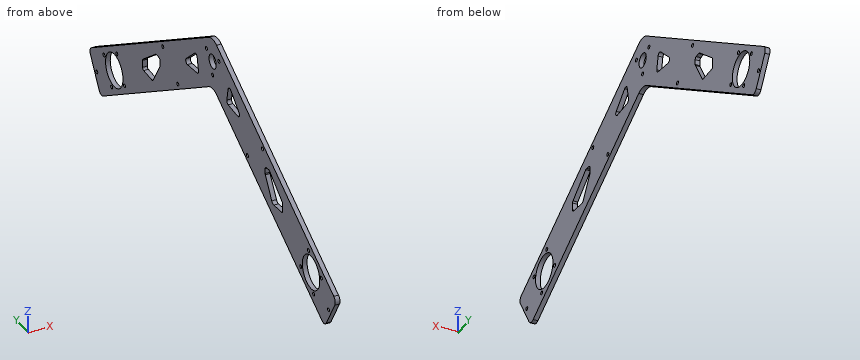
```python
from build123d import *

# Parameters (mm, degrees)
EXTRUDE_BASE_DEPTH         = 3.18
SKETCH4_R                  = 11.5
CUT_MOTOR_HOLES_DEPTH      = 3.18
SKETCH5_R                  = 1.25
MOTOR_SUPPORT_HOLES_DEPTH  = 3.18
SKETCH6_R                  = 1.25
SKETCH6_R_2                = 4.765
SUPPORT_HOLES_DEPTH        = 3.18
CUT_LIGHTENING_HOLES_DEPTH = 3.18


with BuildPart() as part:
    # bogie base → extrude-base (new body)
    with BuildSketch(Plane.YZ):
        with BuildLine():
            Line((-31.39506552, -5.945574909), (-20.11035906, -24.830897255))
            ThreePointArc((-20.11035906, -24.830897255), (-17.653836276, -26.657938255), (-14.624899277, -26.212827416))
            Line((-14.624899277, -26.212827416), (124.870587973, 57.141091427))
            ThreePointArc((124.870587973, 57.141091427), (130, 58.556853997), (135.129412027, 57.141091427))
            Line((135.129412027, 57.141091427), (274.624899277, -26.212827416))
            ThreePointArc((274.624899277, -26.212827416), (277.653836276, -26.657938255), (280.11035906, -24.830897255))
            Line((280.11035906, -24.830897255), (291.39506552, -5.945574909))
            ThreePointArc((291.39506552, -5.945574909), (291.840176358, -2.91663791), (290.013135359, -0.460115126))
            Line((290.013135359, -0.460115126), (135.129412027, 92.088866631))
            ThreePointArc((135.129412027, 92.088866631), (130, 93.504629201), (124.870587973, 92.088866631))
            Line((124.870587973, 92.088866631), (-30.013135359, -0.460115126))
            ThreePointArc((-30.013135359, -0.460115126), (-31.840176358, -2.91663791), (-31.39506552, -5.945574909))
        make_face()
    extrude(amount=EXTRUDE_BASE_DEPTH)

    # Sketch4 → Cut-motor holes (cut)
    with BuildSketch(Plane.YZ):
        with Locations((260, 0)):
            Circle(SKETCH4_R)
        Circle(SKETCH4_R)
    extrude(amount=CUT_MOTOR_HOLES_DEPTH, mode=Mode.SUBTRACT)

    # Sketch5 → motor support holes (cut)
    with BuildSketch(Plane.YZ):
        with Locations((3.419410151, 13.575994778)):
            Circle(SKETCH5_R)
        with Locations((-3.41941001, -13.575994814)):
            Circle(SKETCH5_R)
        with Locations((13.577380102, -3.419759)):
            Circle(SKETCH5_R)
        with Locations((-13.57737996, 3.419758964)):
            Circle(SKETCH5_R)
        with Locations((273.57737996, 3.419758964)):
            Circle(SKETCH5_R)
        with Locations((246.422619898, -3.419759)):
            Circle(SKETCH5_R)
        with Locations((263.41941001, -13.575994814)):
            Circle(SKETCH5_R)
        with Locations((256.580589849, 13.575994778)):
            Circle(SKETCH5_R)
    extrude(amount=MOTOR_SUPPORT_HOLES_DEPTH, mode=Mode.SUBTRACT)

    # Sketch6 → support holes (cut)
    with BuildSketch(Plane.YZ):
        with Locations((64.164835578, 52.110380567)):
            Circle(SKETCH6_R)
        with Locations((84.016579298, 36.433714107)):
            Circle(SKETCH6_R)
        with Locations((130, 77.68)):
            Circle(SKETCH6_R_2)
        with Locations((130, 68.17)):
            Circle(SKETCH6_R)
        with Locations((121.77231361, 82.449200841)):
            Circle(SKETCH6_R)
        with Locations((138.248750332, 82.43704307)):
            Circle(SKETCH6_R)
        with Locations((175.983420702, 36.433714107)):
            Circle(SKETCH6_R)
        with Locations((195.835164422, 52.110380567)):
            Circle(SKETCH6_R)
        with Locations((-23.022924787, -13.757083057)):
            Circle(SKETCH6_R)
        with Locations((283.022924787, -13.757083057)):
            Circle(SKETCH6_R)
    extrude(amount=SUPPORT_HOLES_DEPTH, mode=Mode.SUBTRACT)

    # Sketch7 → Cut-lightening holes (cut)
    with BuildSketch(Plane.YZ):
        with BuildLine():
            Line((54.884000108, 41.646401467), (38.03439682, 28.860792879))
            ThreePointArc((38.03439682, 28.860792879), (37.597600164, 28.332915929), (37.441118366, 27.665863577))
            Line((37.441118366, 27.665863577), (37.441118366, 22.734591544))
            ThreePointArc((37.441118366, 22.734591544), (37.849837551, 21.705462697), (38.853259944, 21.237166789))
            Line((38.853259944, 21.237166789), (49.165938422, 20.63209087))
            ThreePointArc((49.165938422, 20.63209087), (50.727348318, 20.966140733), (51.896208282, 22.053962665))
            Line((51.896208282, 22.053962665), (60.398420976, 35.861757183))
            ThreePointArc((60.398420976, 35.861757183), (60.564389902, 36.239537563), (60.621144468, 36.64824604))
            Line((60.621144468, 36.64824604), (60.621144468, 40.036157787))
            ThreePointArc((60.621144468, 40.036157787), (60.245516663, 41.02902594), (59.306761578, 41.524628912))
            Line((59.306761578, 41.524628912), (55.976338764, 41.939943289))
            ThreePointArc((55.976338764, 41.939943289), (55.401440776, 41.900078528), (54.884000108, 41.646401467))
        make_face()
        with BuildLine():
            Line((200.693238422, 41.524628912), (204.023661236, 41.939943289))
            ThreePointArc((204.023661236, 41.939943289), (204.598559224, 41.900078528), (205.115999892, 41.646401467))
            Line((205.115999892, 41.646401467), (221.96560318, 28.860792879))
            ThreePointArc((221.96560318, 28.860792879), (222.402399836, 28.332915929), (222.558881634, 27.665863577))
            Line((222.558881634, 27.665863577), (222.558881634, 22.734591544))
            ThreePointArc((222.558881634, 22.734591544), (222.150162449, 21.705462697), (221.146740056, 21.237166789))
            Line((221.146740056, 21.237166789), (209.939024731, 20.579576362))
            ThreePointArc((209.939024731, 20.579576362), (209.158319783, 20.746601293), (208.573889801, 21.290512259))
            Line((208.573889801, 21.290512259), (199.601579024, 35.861757183))
            ThreePointArc((199.601579024, 35.861757183), (199.435610098, 36.239537563), (199.378855532, 36.64824604))
            Line((199.378855532, 36.64824604), (199.378855532, 40.036157787))
            ThreePointArc((199.378855532, 40.036157787), (199.754483337, 41.02902594), (200.693238422, 41.524628912))
        make_face()
        with BuildLine():
            Line((106.261574004, 70.658830934), (95.113053624, 60.737670596))
            ThreePointArc((95.113053624, 60.737670596), (94.605778471, 58.452426038), (96.614841284, 57.251036263))
            Line((96.614841284, 57.251036263), (109.502121723, 58.364828314))
            ThreePointArc((109.502121723, 58.364828314), (110.928310049, 59.155267125), (111.292040735, 60.744765992))
            Line((111.292040735, 60.744765992), (109.553280676, 69.552134278))
            ThreePointArc((109.553280676, 69.552134278), (108.22850953, 71.060494424), (106.261574004, 70.658830934))
        make_face()
        with BuildLine():
            Line((148.707959265, 60.744765992), (150.446719324, 69.552134278))
            ThreePointArc((150.446719324, 69.552134278), (151.77149047, 71.060494424), (153.738425996, 70.658830934))
            Line((153.738425996, 70.658830934), (164.886946376, 60.737670596))
            ThreePointArc((164.886946376, 60.737670596), (165.394221529, 58.452426038), (163.385158716, 57.251036263))
            Line((163.385158716, 57.251036263), (150.497878277, 58.364828314))
            ThreePointArc((150.497878277, 58.364828314), (149.071689951, 59.155267125), (148.707959265, 60.744765992))
        make_face()
    extrude(amount=CUT_LIGHTENING_HOLES_DEPTH, mode=Mode.SUBTRACT)


solid = part.part
```
Check sheet for the modelled part. Datum: model origin and axes. Units: mm. Coordinates: 2 decimals unless noted, no trailing zeros. Order: outer loops, then holes, each group sorted by start corner. A loop starts at its lowest first (then second) coordinate and runs counter-clockwise, first axis right, second up. Notation, with made-up numbers: (65, -9.5) -> (70, -9.5) arc R13 cw to (70, 11.5) -> close; hole circle Ø5 at (-4, -27.5). An arc over 180 degrees is marked (long way). Write item = value, one per line. Start each with the question number.
1) Material ranges on L1, parallel to Y at x = 2.05, z = 66.5; L2, parallel to Y at x = 2.05, z = 36; L3, parallel to Y at x = 1, z = -18.5, recorded low to high.
2) Cross-section at B-B (x = 2.35). State how many separate pieces and enclosed holes the cut face has, then the cut area to 3 significant figures.
3) Go/stop test with flat-tipped pins: P1, Ø1.5, axis at x = 2.5, z = 38, coming from the -Y side; P2, Ø2, axis at y = 13.58, z = -3.42, coming from the +X side; P3, Ø1, axis at x = 2, z = 39, coming from the -Y side; P4, Ø1, axis at x = 3, y = 129.5, coming from the -Z side. Record where each tip stops, or that it passes through.
4) Cross-section at A-A (z = 77.68). Enter the section's corners in (x, y) (3 decimals).
Ans:
q1.L1 = 82.05 to 101.59, 110.16 to 149.84, 158.41 to 177.95
q1.L2 = 31 to 47.44, 60.47 to 82.84, 85.19 to 89.49, 170.51 to 174.81, 177.16 to 199.53, 212.56 to 229
q1.L3 = -23.89 to -1.72, 261.72 to 283.89
q2.separate_pieces = 1
q2.enclosed_holes = 24
q2.area = 9,020 mm²
q3.P1 = 33.1
q3.P2 = through
q3.P3 = 35.19
q3.P4 = 58.51
q4.outline = (0, 100.757) -> (3.18, 100.757) -> (3.18, 125.235) -> (0, 125.235) -> close; (0, 134.765) -> (3.18, 134.765) -> (3.18, 159.243) -> (0, 159.243) -> close
